Check sheet for the modelled part. Datum: model origin and axes. Units: mm. Face numbers are marked on the shaded views. A direction names the side the tool comes from. Give positions to 0.01 mm unless a question says otherwise; leave off trailing zeros. Write each loop counter-clockwise with the first axis right and the second up, starting at its lowest first coordinate (ties: lowest second). Pieces come first, ordered by that corner, then holes. Notation, with made-up numbers: M 9,55.25 L 37,55.25 A15 ccw 37,72.25 Z; hole C 57,-14 d3. An arc over 180 degrees is marked long. Write item = value, one per line. Start each with the question number.
1) Sectioned sample at C-C, the plane z = -5.75. Count the separate pieces of the cut face and the enclosed holes in it, then the cut area to 3 significant figures.
2) Gauge pin test, flat ends, axial feed: pin 1 (1 mm diameter, centred on x = -4.5, z = 4, fed in from -Y); pin 2 (1.5 mm diameter, centred on y = 2, z = 3, fed in from -X). Record the tip position at first contact, or that the pin passes through.
3) Set-up check for the marked faces 3 and 4: record each of +Z, -Z, +X, -X, +Y, -Y from which the full face is reachable in a straight line by a thin tool's end or side.
4) Sectioned sample at B-B, the plane z = 0. Record the cut outline in (x, y), then the cut area to 3 significant figures.
5) Sectioned sample at A-A, the plane x = 0. Record the cut outline in (y, z), then the cut area to 3 significant figures.
6) Draft check along X on the marked faces 1 and 2. Enter one of: pulls with the +X half, pulls with the -X half, needs draft (parallel to the pull), parting line crosses it, or undercut.
7) Scan lines: L1, parallel to Z at x = -6.5, y = 0.9; L2, parallel to X at y = 1.55, z = -6; L3, parallel to X at y = 1.55, z = 0. Record each from-to range of solid material in increasing order.
from build123d import *

# Parameters (mm, degrees)
SKETCH1_R           = 12
SKETCH1_R_2         = 1.65
BOSS_EXTRUDE1_DEPTH = 2.5
SKETCH2_R           = 2.1
CUT_EXTRUDE1_DEPTH  = 1.9
CHAMFER1_SIZE       = 1.5
FILLET1_R           = 0.5


with BuildPart() as part:
    # Sketch1 → Boss-Extrude1 (new body)
    with BuildSketch(Plane(origin=(0, 0, 0), x_dir=(1, 0, 0), z_dir=(0, 1, 0))):
        with Locations(Location((0, 0, 0), (0, 0, 270))):
            Circle(SKETCH1_R)
        with Locations(Location((-5.656854249, 5.656854249, 0), (0, 0, 270))):
            Circle(SKETCH1_R_2, mode=Mode.SUBTRACT)
        with Locations(Location((5.656854249, 5.656854249, 0), (0, 0, 270))):
            Circle(SKETCH1_R_2, mode=Mode.SUBTRACT)
        with Locations(Location((5.656854249, -5.656854249, 0), (0, 0, 270))):
            Circle(SKETCH1_R_2, mode=Mode.SUBTRACT)
        with Locations(Location((-5.656854249, -5.656854249, 0), (0, 0, 270))):
            Circle(SKETCH1_R_2, mode=Mode.SUBTRACT)
    extrude(amount=BOSS_EXTRUDE1_DEPTH)

    # Sketch2 → Cut-Extrude1 (cut)
    with BuildSketch(Plane(origin=(0, 2.5, 0), x_dir=(1, 0, 0), z_dir=(0, 1, 0))):
        with Locations(Location((0, 0, 0), (0, 0, 270))):
            Circle(SKETCH2_R)
    extrude(amount=-CUT_EXTRUDE1_DEPTH, mode=Mode.SUBTRACT)

    # Chamfer1
    chamfer1_edges = [part.edges().sort_by_distance(p)[0] for p in [
        (5.656854249, 0, 4.006854249),
        (-5.656854249, 0, 4.006854249),
        (-5.656854249, 0, -7.306854249),
        (5.656854249, 0, -7.306854249),
    ]]
    chamfer(chamfer1_edges, length=CHAMFER1_SIZE)

    # Fillet1
    fillet1_edges = [part.edges().sort_by_distance(p)[0] for p in [
        (0, 0, -12),
        (0, 2.5, -12),
    ]]
    fillet(fillet1_edges, radius=FILLET1_R)


solid = part.part
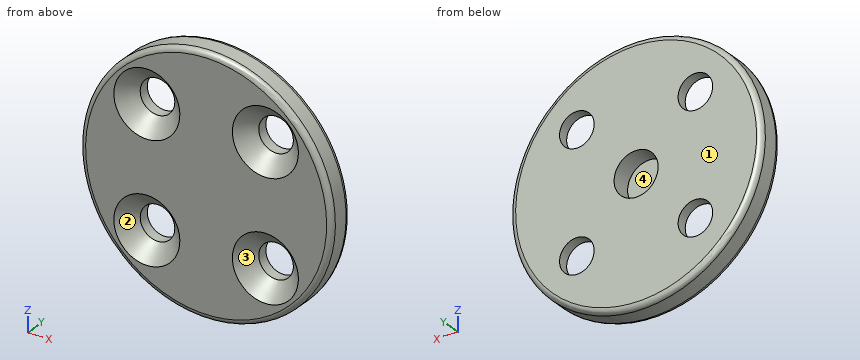
Data:
q1.separate_pieces = 3
q1.enclosed_holes = 0
q1.area = 31.4 mm2
q2.pin_1 = 0.63
q2.pin_2 = -11.79
q3.face_3 = -Y
q3.face_4 = +Y
q4.outline = M -12,0.5 A0.5 ccw -11.5,0 L 11.5,0 A0.5 ccw 12,0.5 L 12,2 A0.5 ccw 11.5,2.5 L 2.1,2.5 L 2.1,0.6 L -2.1,0.6 L -2.1,2.5 L -11.5,2.5 A0.5 ccw -12,2 Z
q4.area = 51.8 mm2
q5.outline = M 0,-11.5 A0.5 ccw 0.5,-12 L 2,-12 A0.5 ccw 2.5,-11.5 L 2.5,-2.1 L 0.6,-2.1 L 0.6,2.1 L 2.5,2.1 L 2.5,11.5 A0.5 ccw 2,12 L 0.5,12 A0.5 ccw 0,11.5 Z
q5.area = 51.8 mm2
q6.face_1 = needs draft
q6.face_2 = undercut
q7.L1 = -10.09 to -7.74, -3.57 to 3.57, 7.74 to 10.09
q7.L2 = -10.39 to -7.27, -4.04 to 4.04, 7.27 to 10.39
q7.L3 = -12 to -2.1, 2.1 to 12
